from build123d import *

# Parameters (mm, degrees)
SKETCH1_W           = 124
SKETCH1_H           = 70
BOSS_EXTRUDE1_DEPTH = 10
SKETCH11_R          = 2.15
CUT_EXTRUDE4_DEPTH  = 79.938779664
SKETCH17_R          = 3.75
CUT_EXTRUDE5_DEPTH  = 4


with BuildPart() as part:
    # Sketch1 → Boss-Extrude1 (new body)
    with BuildSketch(Plane(origin=(0, 0, 0), x_dir=(1, 0, 0), z_dir=(0, 1, 0))):
        with Locations((3.263157895, -8.267206478)):
            Rectangle(SKETCH1_W, SKETCH1_H)
    extrude(amount=BOSS_EXTRUDE1_DEPTH)

    # Sketch11 → Cut-Extrude4 (cut, through all)
    with BuildSketch(Plane(origin=(0, 10, 0), x_dir=(1, 0, 0), z_dir=(0, 1, 0))):
        with Locations(Location((-50.736842105, 18.732793522, 0), (0, 0, 270))):
            Circle(SKETCH11_R)
        with Locations(Location((-40.736842105, 18.732793522, 0), (0, 0, 270))):
            Circle(SKETCH11_R)
        with Locations(Location((-50.736842105, -35.267206478, 0), (0, 0, 270))):
            Circle(SKETCH11_R)
        with Locations(Location((-40.736842105, -35.267206478, 0), (0, 0, 270))):
            Circle(SKETCH11_R)
        with Locations(Location((47.263157895, 18.732793522, 0), (0, 0, 270))):
            Circle(SKETCH11_R)
        with Locations(Location((57.263157895, 18.732793522, 0), (0, 0, 270))):
            Circle(SKETCH11_R)
        with Locations(Location((47.263157895, -35.267206478, 0), (0, 0, 270))):
            Circle(SKETCH11_R)
        with Locations(Location((57.263157895, -35.267206478, 0), (0, 0, 270))):
            Circle(SKETCH11_R)
    extrude(amount=-CUT_EXTRUDE4_DEPTH, mode=Mode.SUBTRACT)

    # Sketch17 → Cut-Extrude5 (cut)
    with BuildSketch(Plane(origin=(0, 10, 0), x_dir=(1, 0, 0), z_dir=(0, 1, 0))):
        with Locations(Location((-50.736842105, 18.732793522, 0), (0, 0, 270))):
            Circle(SKETCH17_R)
        with Locations(Location((-40.736842105, 18.732793522, 0), (0, 0, 270))):
            Circle(SKETCH17_R)
        with Locations(Location((47.263157895, 18.732793522, 0), (0, 0, 270))):
            Circle(SKETCH17_R)
        with Locations(Location((57.263157895, 18.732793522, 0), (0, 0, 270))):
            Circle(SKETCH17_R)
        with Locations(Location((57.263157895, -35.267206478, 0), (0, 0, 270))):
            Circle(SKETCH17_R)
        with Locations(Location((47.263157895, -35.267206478, 0), (0, 0, 270))):
            Circle(SKETCH17_R)
        with Locations(Location((-40.736842105, -35.267206478, 0), (0, 0, 270))):
            Circle(SKETCH17_R)
        with Locations(Location((-50.736842105, -35.267206478, 0), (0, 0, 270))):
            Circle(SKETCH17_R)
    extrude(amount=-CUT_EXTRUDE5_DEPTH, mode=Mode.SUBTRACT)


solid = part.part
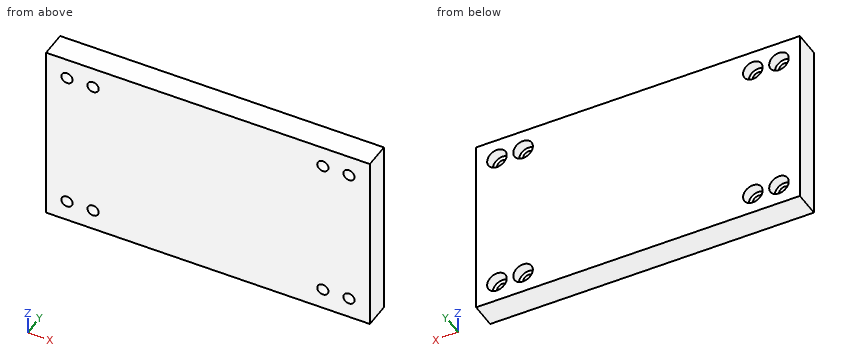
Work out the finished part from the listing and answer in its coordinate system (mm). Round coordinates to 2 decimals unless told otherwise and drop trailing zeros. Answer in a Markdown table with one row per item. Add a question column.
1. Find the intervals of material crossed by line 1 along X through (y, z) = (5.25, -20.5), in increasing order. Write a range as from..to.
2. Given pin 1 (1 mm diameter, centred on x = 50, z = -19.5, fed in from +Y), flat-ended and moving along its own axis, determine where the tip first touches the part or whether it passes through.
3. A cutting plane is placed at A-A, the plane y = 7.5. Count the separate pieces of the cut face and the enclosed holes in it, and give its area (3 significant figures).
Worked out:
| question | item | result |
|---|---|---|
| 1 | line 1 | -58.74..-51.96, -49.51..-41.96, -39.51..46.04, 48.49..56.04, 58.49..65.26 |
| 2 | pin 1 | y = 6 |
| 3 | separate pieces | 1 |
| 3 | enclosed holes | 8 |
| 3 | area | 8,330 mm^2 |
